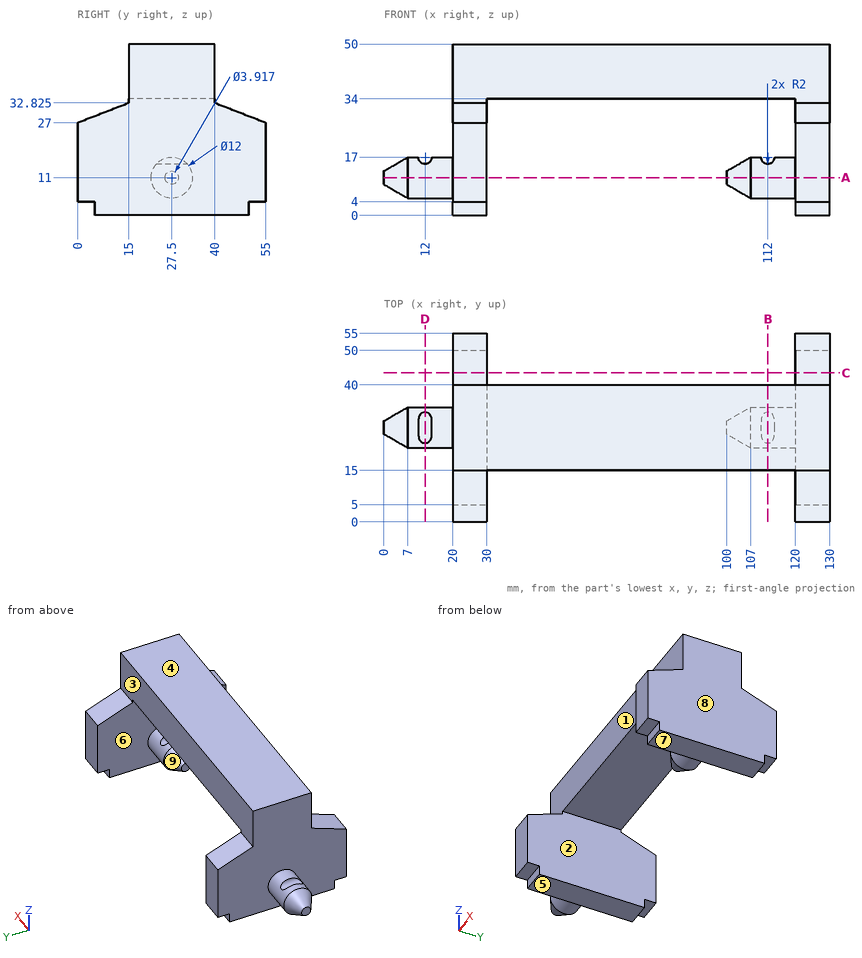
Job drawing, mm, ordinate dimensions from the low corner. One solid piece. A direction names the side the tool comes from. Coordinates: 2 decimals unless noted, no trailing zeros. Write each loop counter-clockwise with the first axis right and the second up, starting at its lowest first coordinate (ties: lowest second). Pieces come first, ordered by that corner, then holes.
Item 1: Pin check, flat tips, straight feed: pin 1 (10 mm diameter, centred on y = 17, z = 19, fed in from -X); pin 2 (4 mm diameter, centred on x = 126, y = 52.5, fed in from -Z); pin 3 (3 mm diameter, centred on x = 47, z = 38.5, fed in from +Y); pin 4 (10 mm diameter, centred on x = 38, z = 19, fed in from -Y). Stop position of each tip, or through.
Item 2: Slice it at A-A (z = 11). Write the cut outline in (x, y).
Item 3: Probe line 1 (X direction, y = 42, z = 12.5); line 2 (X direction, y = 26.5, z = 16); line 3 (Z direction, x = 70, y = 30.5). List the from-to ranges inside material, lowest first.
Item 4: Slice it at C-C (y = 43.5). Write the cut outline in (x, z).
Item 5: Which spindle directions (+Z, -Z, +X, -X, +Y, -Y) get a long thin tool onto all of the face, cutting with end or side? Do the marked faces 1, 2, 3, 4 and 5. Say none if no direction does.
Item 6: Slice it at D-D (x = 12). Write the cut outline in (y, z), and give its area (3 significant figures).
Item 7: Mould opens along X. For the marked faces 6, 7, 8 and 9 say: released by +X, released by -X, zero draft, split by the parting line, or undercut.
Item 8: Slice it at B-B (x = 112). Write the cut outline in (y, z), and give its area (3 significant figures).
Results found:
1. pin 1: stops at x = 20
1. pin 2: stops at z = 4
1. pin 3: stops at y = 40
1. pin 4: passes through
2. outline: (0, 25.54) - (7, 21.5) - (20, 21.5) - (20, 0) - (30, 0) - (30, 55) - (20, 55) - (20, 33.5) - (7, 33.5) - (0, 29.46) - close; (100, 25.54) - (107, 21.5) - (120, 21.5) - (120, 0) - (130, 0) - (130, 55) - (120, 55) - (120, 33.5) - (107, 33.5) - (100, 29.46) - close
3. line 1: x = 20 to 30, 120 to 130
3. line 2: x = 5.44 to 10.27, 13.73 to 30, 105.44 to 110.27, 113.73 to 130
3. line 3: z = 34 to 50
4. outline: (20, 0) - (30, 0) - (30, 31.47) - (20, 31.47) - close; (120, 0) - (130, 0) - (130, 31.47) - (120, 31.47) - close
5. face 1: +Z, +X, -X, -Y
5. face 2: -Z, +Y, -Y
5. face 3: +Z, +X, -X, +Y
5. face 4: +Z, +X, -X, +Y, -Y
5. face 5: -Z, +X, -X, +Y, -Y
6. outline: (23.03, 15) arc R6 ccw (long way) to (31.97, 15) - close
6. area: 101 mm2
7. face 6: undercut
7. face 7: zero draft
7. face 8: released by +X
7. face 9: undercut
8. outline: (15, 34) - (40, 34) - (40, 50) - (15, 50) - close; (23.03, 15) arc R6 ccw (long way) to (31.97, 15) - close
8. area: 501 mm2
